Can you work these out from the drawing? Everything is in mm from the part's minimum corner. Coordinates: 2 decimals unless noted, no trailing zeros. Order: outer loops, then holes, each group sorted by start corner. A loop starts at its lowest first (then second) coordinate and runs counter-clockwise, first axis right, second up. Notation, with made-up numbers: (60.25, 3) - (83.25, 3) arc R15 ccw to (83.25, 9) - close; hole circle Ø6 at (-38, 67.5). An arc over 180 degrees is marked (long way). Answer as CSV lines item,"result". Start each with the question number.
Q1. Thinking about a two-plate mould opening in Y: for the marked faces 1, 2, 3 and 4, which applies, released by +Y, released by -Y, zero draft, split by the parting line, or undercut?
Q2. For pin 1 Ø8 at (x, z) = (28.5, 5) entering from -Y; pin 2 Ø3 at (y, z) = (14, 5) entering from -X; pin 3 Ø10 at (x, z) = (28.5, 7) entering from -Y, each with a flat end and sliding along its axis, tell me the tip position at first contact or that it passes through.
Q3. I need wall thicknesses on line 1 (Z direction, x = 6, y = 58); line 2 (Y direction, x = 29, z = 9.5); line 3 (Y direction, x = 25.5, z = 9). Which ranges of each line are inside material? Lowest first, please.
Q4. Suppose I cut it at B-B (y = 45). Please give me the cut outline in (x, z), then the cut area to 3 significant figures.
Q5. Suppose I cut it at A-A (x = 81). Please give me the cut outline in (y, z), then the cut area to 3 significant figures.
Q6. Suppose I cut it at C-C (z = 10.25). Please give me the cut outline in (x, y).
Q7. Suppose I cut it at D-D (z = 3.5). Please give me the cut outline in (x, y).
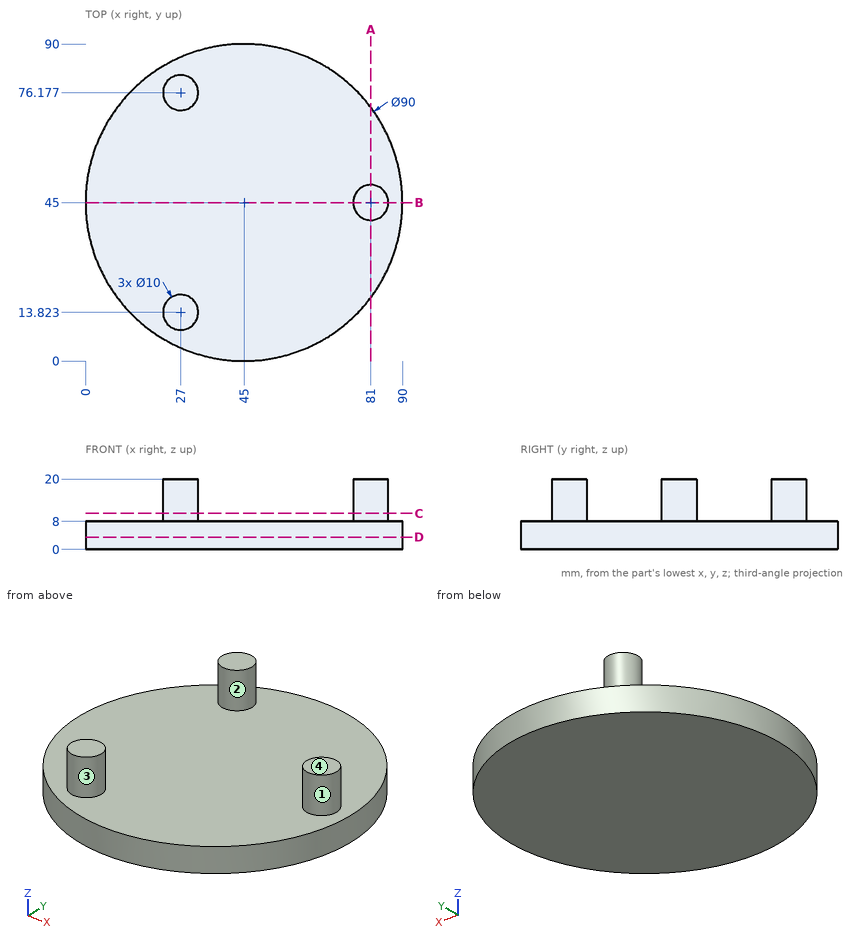
Here are the results:
1,face 1,"split by the parting line"
1,face 2,"undercut"
1,face 3,"undercut"
1,face 4,"zero draft"
2,pin 1,"stops at y = 1.77"
2,pin 2,"stops at x = 11.02"
2,pin 3,"stops at y = 1.49"
3,line 1,"z = 0 to 8"
3,line 2,"y = 9.24 to 18.41, 71.59 to 80.76"
3,line 3,"y = 9.05 to 18.59, 71.41 to 80.95"
4,outline,"(0, 0) - (90, 0) - (90, 8) - (86, 8) - (86, 20) - (76, 20) - (76, 8) - (0, 8) - close"
4,area,"840 mm²"
5,outline,"(18, 0) - (72, 0) - (72, 8) - (50, 8) - (50, 20) - (40, 20) - (40, 8) - (18, 8) - close"
5,area,"552 mm²"
6,outline,"circle Ø10 at (27, 13.82); circle Ø10 at (27, 76.18); circle Ø10 at (81, 45)"
7,outline,"circle Ø90 at (45, 45)"
